Geometry check sheet. Reference: the model listing, model coordinates, mm. A direction names the side the tool comes from. Coordinates: 2 decimals unless noted, no trailing zeros. Order: outer loops, then holes, each group sorted by start corner. A loop starts at its lowest first (then second) coordinate and runs counter-clockwise, first axis right, second up. Notation, with made-up numbers: (72.5, 54) - (102.5, 54) arc R15 cw to (102.5, 62) - close; hole circle Ø6 at (-7, 66). An arc over 180 degrees is marked (long way). Use CSV: the item, a comma, the result in double quotes. Start each with the question number.
1) Sectioned sample at A-A, the plane z = 46.5. Record the cut outline in (x, y).
2) Depth check by flat-ended pin: P1, Ø0.8, axis at y = 49.5, z = 52, coming from the -X side; P2, Ø0.8, axis at x = 25, y = 49.5, coming from the -Z side; P3, Ø5, axis at x = 26.5, y = 12, coming from the +Z side. Enter the tip coordinate at first touch or a pass-through.
3) Sectioned sample at B-B, the plane x = 10.5. Record the cut outline in (y, z), and give its area (3 significant figures).
4) Sectioned sample at C-C, the plane y = 25. Record the cut outline in (x, z).
5) Thickness scan on probe 1 along Z at (x, y) = (34.5, 21.5); probe 2 along Y at (x, z) = (45, 21); probe 3 along Z at (x, y) = (17.5, 13). Record the ranges inside material, lowest first. Write a range as [from, to].
6) Draft check along Z on faces 4 (the flat face through (25, 25, 36)), 5 (the flat face through (24.671, 32.823, 42.267)), 6 (the flat face through (24.7, 0.7, 0.8)), 7 (the flat face through (25, 36, 47)). Enter one of: released by +Z, released by -Z, zero draft, split by the parting line, or undercut.
7) Tool access check on faces 1 (the flat face through (24.65, 17.267, 17.177)), 2 (the flat face through (0.8, 13.3, 46.6)), 3 (the flat face through (49.26, 16.51, 41.86)). Record the directions out of +Z, -Z, +X, -X, +Y, -Y that give a thin tool (end or side, any length) a straight path to the whole face; none if there is none.
8) Sectioned sample at D-D, the plane z = 26.5. Record the cut outline in (x, y), and give its area (3 significant figures).
from build123d import *

# Parameters (mm, degrees)
SKETCH1_W                = 50
SKETCH1_H                = 50
BOSS_EXTRUDE1_DEPTH      = 50
CUT_EXTRUDE1_DEPTH       = 87.602540378
CHAMFER1_SIZE            = 1.5
BOSS_EXTRUDE2_DEPTH      = 7
BOSS_EXTRUDE2_DEPTH_BACK = 10
SKETCH3_W                = 7
SKETCH3_H                = 1
SKETCH4_W                = 1.8
SKETCH4_H                = 1.8
CUT_EXTRUDE2_DEPTH       = 7


with BuildPart() as part:
    # Sketch1 → Boss-Extrude1 (new body)
    with BuildSketch(Plane.XY):
        with Locations((25, 25)):
            Rectangle(SKETCH1_W, SKETCH1_H)
    extrude(amount=BOSS_EXTRUDE1_DEPTH)

    # Sketch2 → Cut-Extrude1 (cut, through all)
    with BuildSketch(Plane.ZY):
        Polygon((36, 29.556349186), (29.556349186, 36), (20.443650814, 36), (14, 29.556349186), (14, 20.443650814), (20.443650814, 14), (29.556349186, 14), (36, 20.443650814), align=None)
        Polygon((54.556349186, 36), (45.443650814, 36), (39, 29.556349186), (39, 20.443650814), (45.443650814, 14), (54.556349186, 14), (61, 20.443650814), (61, 29.556349186), align=None)
    extrude(amount=-CUT_EXTRUDE1_DEPTH, mode=Mode.SUBTRACT)

    # Chamfer1
    chamfer1_edges = [part.edges().sort_by_distance(p)[0] for p in [
        (50, 7, 50),
        (0, 7, 50),
        (50, 43, 50),
        (25, 36, 50),
        (25, 14, 50),
        (25, 50, 50),
        (50, 14, 47.721825407),
        (50, 36, 47.721825407),
        (0, 14, 47.721825407),
        (0, 36, 47.721825407),
        (0, 32.778174593, 42.221825407),
        (0, 17.221825407, 42.221825407),
        (50, 17.221825407, 42.221825407),
        (50, 32.778174593, 42.221825407),
        (0, 43, 50),
        (25, 50, 0),
        (50, 25, 0),
        (25, 0, 0),
        (0, 25, 0),
        (25, 0, 50),
        (0, 50, 25),
        (50, 50, 25),
        (50, 0, 25),
        (0, 0, 25),
    ]]
    chamfer(chamfer1_edges, length=CHAMFER1_SIZE)

    # Sketch3 → Boss-Extrude2 (add, two sides: drawn at the far end of the back side and taken through both)
    with BuildSketch(Plane.XY.offset(50).offset(-BOSS_EXTRUDE2_DEPTH_BACK)):
        with Locations((25, 49.5)):
            Rectangle(SKETCH3_W, SKETCH3_H)
    extrude(amount=BOSS_EXTRUDE2_DEPTH + BOSS_EXTRUDE2_DEPTH_BACK)

    # Sketch4 → Cut-Extrude2 (cut)
    with BuildSketch(Plane.XZ.offset(-49)):
        with Locations((25, 53.6)):
            Rectangle(SKETCH4_W, SKETCH4_H)
    extrude(amount=-CUT_EXTRUDE2_DEPTH, mode=Mode.SUBTRACT)


solid = part.part
Evaluation:
1,outline,"(0, 1.5) - (1.5, 0) - (48.5, 0) - (50, 1.5) - (50, 12.5) - (48.5, 14) - (1.5, 14) - (0, 12.5) - close; (0, 37.5) - (1.5, 36) - (48.5, 36) - (50, 37.5) - (50, 48.5) - (48.5, 50) - (1.5, 50) - (0, 48.5) - close"
2,P1,"x = 21.5"
2,P2,"z = 0.6"
2,P3,"z = 50"
3,outline,"(0, 1.5) - (1.5, 0) - (48.5, 0) - (50, 1.5) - (50, 48.5) - (48.5, 50) - (37.5, 50) - (36, 48.5) - (36, 45.44) - (29.56, 39) - (20.44, 39) - (14, 45.44) - (14, 48.5) - (12.5, 50) - (1.5, 50) - (0, 48.5) - close; hole (14, 20.44) - (20.44, 14) - (29.56, 14) - (36, 20.44) - (36, 29.56) - (29.56, 36) - (20.44, 36) - (14, 29.56) - close"
3,area,"1,890 mm²"
4,outline,"(0, 1.5) - (1.5, 0) - (48.5, 0) - (50, 1.5) - (50, 14) - (0, 14) - close; (0, 36) - (50, 36) - (50, 39) - (0, 39) - close"
5,probe 1,"[0, 14], [36, 39]"
5,probe 2,"[0, 14], [36, 50]"
5,probe 3,"[0, 49.5]"
6,face 4,"undercut"
6,face 5,"released by +Z"
6,face 6,"released by -Z"
6,face 7,"zero draft"
7,face 1,"+X, -X"
7,face 2,"+Z, -X"
7,face 3,"+Z, +X"
8,outline,"(0, 1.5) - (1.5, 0) - (48.5, 0) - (50, 1.5) - (50, 14) - (0, 14) - close; (0, 36) - (50, 36) - (50, 48.5) - (48.5, 50) - (1.5, 50) - (0, 48.5) - close"
8,area,"1,400 mm²"
